Geometry: final body of the model. Coordinates: model frame, mm. Face numbers are marked on the shaded views. A direction names the side the tool comes from. Coordinates: 2 decimals unless noted, no trailing zeros. Order: outer loops, then holes, each group sorted by start corner. A loop starts at its lowest first (then second) coordinate and runs counter-clockwise, first axis right, second up. Notation, with made-up numbers: (33.5, 78.25) -> (54.5, 78.25) arc R25 ccw to (54.5, 109.25) -> close; hole circle Ø10 at (-26, 15.5). An arc over 180 degrees is marked (long way). Use one line per item in the form item = value.
```python
from build123d import *

# Parameters (mm, degrees)
SKETCH1_W           = 14.5
SKETCH1_H           = 21.5
BOSS_EXTRUDE1_DEPTH = 6
SHELL1_T            = 2
SKETCH3_W           = 2
SKETCH3_H           = 14.5
BOSS_EXTRUDE3_DEPTH = 2
SKETCH4_W           = 5
SKETCH4_H           = 5
CUT_EXTRUDE1_DEPTH  = 2
FILLET1_R           = 1


with BuildPart() as part:
    # Sketch1 → Boss-Extrude1 (new body)
    with BuildSketch(Plane(origin=(0, 0, 0), x_dir=(1, 0, 0), z_dir=(0, 1, 0))):
        Rectangle(SKETCH1_W, SKETCH1_H)
    extrude(amount=BOSS_EXTRUDE1_DEPTH)

    # Shell1
    shell1_openings = [part.faces().sort_by_distance(p)[0] for p in [
        (0, 3, 10.75),
        (0, 6, 0),
    ]]
    offset(amount=SHELL1_T, openings=shell1_openings, kind=Kind.INTERSECTION)

    # Sketch3 → Boss-Extrude3 (add)
    with BuildSketch(Plane(origin=(0, 6, 0), x_dir=(1, 0, 0), z_dir=(0, 1, 0))):
        with BuildLine():
            Line((-7.25, 10.75), (-7.25, 3.75))
            Line((-7.25, 3.75), (-5.25, 3.75))
            ThreePointArc((-5.25, 3.75), (0, 9), (5.25, 3.75))
            Line((5.25, 3.75), (7.25, 3.75))
            Line((7.25, 3.75), (7.25, 10.75))
            Line((7.25, 10.75), (-7.25, 10.75))
        make_face()
        with Locations((-6.25, -3.5)):
            Rectangle(SKETCH3_W, SKETCH3_H)
        with Locations((6.25, -3.5)):
            Rectangle(SKETCH3_W, SKETCH3_H)
    extrude(amount=-BOSS_EXTRUDE3_DEPTH)

    # Sketch4 → Cut-Extrude1 (cut)
    with BuildSketch(Plane(origin=(0, 0, 0), x_dir=(1, 0, 0), z_dir=(0, 1, 0))):
        with Locations((-2.25, -3.75)):
            Rectangle(SKETCH4_W, SKETCH4_H)
    extrude(amount=-CUT_EXTRUDE1_DEPTH, mode=Mode.SUBTRACT)

    # Fillet1
    fillet1_edges = [part.edges().sort_by_distance(p)[0] for p in [
        (-9.25, 6, -1),
        (-7.25, 6, 10.75),
        (7.25, 6, 10.75),
        (0, 6, -9),
        (-5.25, 6, 3.5),
        (-6.25, 4, 10.75),
        (-5.25, 5, 10.75),
        (5.25, 5, 10.75),
        (6.25, 4, 10.75),
        (5.25, 6, 3.5),
        (9.25, 6, -1),
        (-9.25, 2, -12.75),
        (9.25, 2, -12.75),
        (0, 6, -12.75),
    ]]
    fillet(fillet1_edges, radius=FILLET1_R - 0.0001)  # a hair under: the kernel refuses the full size


solid = part.part
```
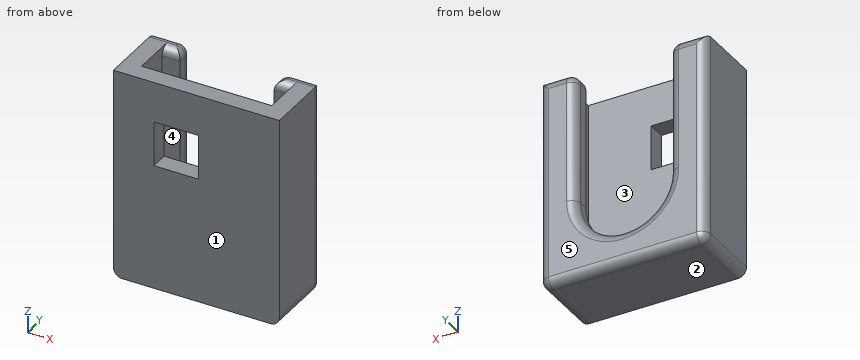
1) Section B-B, the plane x = 0. Output: boundary loops of the cut face in (y, z).
Results found:
outline = (-2, -12.75) -> (5, -12.75) arc R1 ccw to (6, -11.75) -> (6, -10) arc R1 ccw to (5, -9) -> (4, -9) -> (4, -10.75) -> (0, -10.75) -> (0, 1.25) -> (-2, 1.25) -> close; (-2, 6.25) -> (0, 6.25) -> (0, 10.75) -> (-2, 10.75) -> close
2) Section C-C, the plane y = 2. Output: boundary loops of the cut face in (x, z), and give its area (3 significant figures).
Results found:
outline = (-9.25, -11.75) arc R1 ccw to (-8.25, -12.75) -> (8.25, -12.75) arc R1 ccw to (9.25, -11.75) -> (9.25, 10.75) -> (7.25, 10.75) -> (7.25, -10.75) -> (-7.25, -10.75) -> (-7.25, 10.75) -> (-9.25, 10.75) -> close
area = 123 mm2
3) Section D-D, the plane z = 9.25. Output: boundary loops of the cut face in (x, y).
Results found:
outline = (-9.25, -2) -> (9.25, -2) -> (9.25, 5) arc R1 ccw to (8.25, 6) -> (6.25, 6) arc R1 ccw to (5.25, 5) -> (5.25, 4) -> (7.25, 4) -> (7.25, 0) -> (-7.25, 0) -> (-7.25, 4) -> (-5.25, 4) -> (-5.25, 5) arc R1 ccw to (-6.25, 6) -> (-8.25, 6) arc R1 ccw to (-9.25, 5) -> close
4) Pull-direction query (Y, two-part tool) for the marked faces 1, 2 and 3; classes: released by +Y, released by -Y, zero draft, split by the parting line, or undercut.
Results found:
face_1 = released by -Y
face_2 = zero draft
face_3 = undercut
5) Contact query for flat-ended pins moving along their axis: P1, Ø8, axis at x = -5, z = -4.5, coming from the +Y side; P2, Ø4.5, axis at x = -0.5, z = -1, coming from the +Y side. Output: stop coordinate, or through.
Results found:
P1 = 6
P2 = 0
6) Material intervals for probe 1 along X at (y, z) = (-0.25, 5.75); probe 2 along X at (y, z) = (4.5, 4.5); probe 3 along Y at (x, z) = (2.5, 8), sorted ascending. Write a range as from..to.
Results found:
probe_1 = -9.25..-4.75, 0.25..9.25
probe_2 = -9.25..-5.25, 5.25..9.25
probe_3 = -2..0
7) Access query for the marked faces 4 and 5. Directions: +Z, -Z, +X, -X, +Y, -Y. A direction counts if a zero-diameter tool reaches every point of the face in a straight line with its end or side. Return the directions, or none.
Results found:
face_4 = +Z
face_5 = +Z, -Z, +X, -X, +Y
8) Section A-A, the plane z = 4.25. Output: boundary loops of the cut face in (x, y).
Results found:
outline = (-9.25, -2) -> (-4.75, -2) -> (-4.75, 0) -> (-7.25, 0) -> (-7.25, 4) -> (-5.25, 4) -> (-5.25, 5) arc R1 ccw to (-6.25, 6) -> (-8.25, 6) arc R1 ccw to (-9.25, 5) -> close; (0.25, -2) -> (9.25, -2) -> (9.25, 5) arc R1 ccw to (8.25, 6) -> (6.25, 6) arc R1 ccw to (5.25, 5) -> (5.25, 4) -> (7.25, 4) -> (7.25, 0) -> (0.25, 0) -> close
